```python
from build123d import *

# Parameters (mm, degrees)
F1_R          = 1.2
F2_DEPTH      = 2
F3_R          = 2
F4_W          = 4
F4_H          = 4.75
F5_DEPTH      = 9
F6_W          = 8.8
F6_H          = 2
F6_W_2        = 2
F6_H_2        = 6.5
F7_DEPTH      = 4
F8_R          = 0.8
F9_DEPTH      = 4
F10_T4_DEPTH  = 2
F10_S5_R      = 0.8
F10_T6_DEPTH  = 3
F10_T10_DEPTH = 6.5
F10_T15_DEPTH = 6.5
F10_T20_DEPTH = 2
F10_S21_R     = 0.8
F10_T22_DEPTH = 3
F10_T27_DEPTH = 6.5
F10_S29_R     = 0.8
F10_T30_DEPTH = 5
F10_T33_DEPTH = 4.5
F10_T40_DEPTH = 4.5
F10_T44_DEPTH = 6.5
F10_S46_R     = 0.8
F10_T47_DEPTH = 5
F10_T49_DEPTH = 6.5
F10_T51_DEPTH = 11.5
F11_W         = 2
F11_H         = 18
F12_DEPTH     = 12
F13_R         = 1.55
F13_R_2       = 0.8
F14_DEPTH     = 2
F15_R         = 0.8
F16_DEPTH     = 2
F18_W         = 20.8
F18_H         = 21.9
F19_DEPTH     = 0.4


# Not quite as in the source:
# - a fillet or chamfer that OpenCascade refuses, or shapes differently, is made with other operations: its cross-section is extruded or revolved along the edge and cut away or added
# - two fillets or chamfers of one size are made in one step


with BuildPart() as f2:
    # F1 (on Top) → F2 (new body)
    with BuildSketch(Plane.XY):
        with BuildLine():
            Line((-4.2895651858, 24.55), (-9.8, 24.55))
            Line((-9.8, 24.55), (-9.8, 6.55))
            Line((-9.8, 6.55), (-4.3, 6.55))
            Line((-4.3, 6.55), (-4.3, -5))
            ThreePointArc((-4.3, -5), (-3.4213203436, -7.1213203436), (-1.3, -8))
            Line((-1.3, -8), (22.7, -8))
            ThreePointArc((22.7, -8), (24.8213203436, -7.1213203436), (25.7, -5))
            Line((25.7, -5), (25.7, 6.55))
            Line((25.7, 6.55), (31.2, 6.55))
            Line((31.2, 6.55), (31.2, 24.55))
            Line((31.2, 24.55), (25.6895651858, 24.55))
            ThreePointArc((25.6895651858, 24.55), (24.7310096012, 26.5079402166), (22.7, 27.3))
            Line((22.7, 27.3), (-1.3, 27.3))
            ThreePointArc((-1.3, 27.3), (-3.3310096012, 26.5079402166), (-4.2895651858, 24.55))
        make_face()
        with Locations((-1.3, -5)):
            Circle(F1_R, mode=Mode.SUBTRACT)
        with Locations((22.7, -5)):
            Circle(F1_R, mode=Mode.SUBTRACT)
        with Locations((-1.3, 24.3)):
            Circle(F1_R, mode=Mode.SUBTRACT)
        with Locations((22.7, 24.3)):
            Circle(F1_R, mode=Mode.SUBTRACT)
    extrude(amount=F2_DEPTH)

    # F3
    f3_edges = [f2.edges().sort_by_distance(p)[0] for p in [
        (-4.289565, 24.55, 1),
        (-4.3, 6.55, 1),
        (25.7, 6.55, 1),
        (25.689565, 24.55, 1),
    ]]
    fillet(f3_edges, radius=F3_R)

    # F4 (on face) → F5 (join)
    with BuildSketch(Plane(origin=(0, 0, 0), x_dir=(1, 0, 0), z_dir=(0, 0, -1))):
        with Locations((13.8, 2.675)):
            Rectangle(F4_W, F4_H)
        with Locations((13.8, -23.975)):
            Rectangle(F4_W, F4_H)
    extrude(amount=F5_DEPTH)

    # F6 (on face) → F7 (join)
    with BuildSketch(Plane(origin=(0, 0, 0), x_dir=(1, 0, 0), z_dir=(0, 0, -1))):
        Polygon((-2.3, -18.3), (-0.3, -18.3), (-0.3, 0.3), (11.8, 0.3), (11.8, 2.3), (-2.3, 2.3), align=None)
        with Locations((7.4, -22.6)):
            Rectangle(F6_W, F6_H)
        with Locations((21.5, -3.25)):
            Rectangle(F6_W_2, F6_H_2)
    extrude(amount=F7_DEPTH)

    # F8 (on face) → F9 (cut, through all)
    with BuildSketch(Plane.YZ.offset(15.8)):
        with Locations((23.4, -5.75)):
            Circle(F8_R)
        with Locations((-2.1, -5.75)):
            Circle(F8_R)
    extrude(amount=-F9_DEPTH, mode=Mode.SUBTRACT)

    # F10: fillet of radius 1 on 10 edges, made by hand


with BuildPart() as f10_tool2:
    # F10_s3 → F10_t4 (new body)
    with BuildSketch(Plane.XZ.offset(0.3)):
        with BuildLine():
            ThreePointArc((11.8, -5), (11.5071067812, -4.2928932188), (10.8, -4))
            Line((10.8, -4), (11.8, -4))
            Line((11.8, -4), (11.8, -5))
        make_face()
    extrude(amount=F10_T4_DEPTH)

    # F10_s5 → F10_t6 (cut, symmetric)
    with BuildSketch(Plane.YZ.offset(11.3)):
        with Locations((-2.1, -5.75)):
            Circle(F10_S5_R)
    extrude(amount=F10_T6_DEPTH, both=True, mode=Mode.SUBTRACT)


with BuildPart() as f2_1:
    add(f2.part)

    # F10_t1: union F10_tool2
    add(f10_tool2.part)


with BuildPart() as f10_tool8:
    # F10_s9 → F10_t10 (new body)
    with BuildSketch(Plane.XY.offset(2.5)):
        with BuildLine():
            ThreePointArc((11.8, -3.3), (11.5071067812, -2.5928932188), (10.8, -2.3))
            Line((10.8, -2.3), (11.8, -2.3))
            Line((11.8, -2.3), (11.8, -3.3))
        make_face()
    extrude(amount=-F10_T10_DEPTH)

    split(bisect_by=Plane.XY.offset(2), keep=Keep.BOTTOM)


with BuildPart() as f2_2:
    add(f2_1.part)

    # F10_t7: union F10_tool8
    add(f10_tool8.part)


with BuildPart() as f10_tool13:
    # F10_s14 → F10_t15 (new body)
    with BuildSketch(Plane.XY.offset(2.5)):
        with BuildLine():
            ThreePointArc((11.8, 24.6), (11.5071067812, 23.8928932188), (10.8, 23.6))
            Line((10.8, 23.6), (11.8, 23.6))
            Line((11.8, 23.6), (11.8, 24.6))
        make_face()
    extrude(amount=-F10_T15_DEPTH)

    split(bisect_by=Plane.XY.offset(2), keep=Keep.BOTTOM)


with BuildPart() as f2_3:
    add(f2_2.part)

    # F10_t12: union F10_tool13
    add(f10_tool13.part)


with BuildPart() as f10_tool18:
    # F10_s19 → F10_t20 (new body)
    with BuildSketch(Plane.XZ.offset(-23.6)):
        with BuildLine():
            ThreePointArc((11.8, -5), (11.5071067812, -4.2928932188), (10.8, -4))
            Line((10.8, -4), (11.8, -4))
            Line((11.8, -4), (11.8, -5))
        make_face()
    extrude(amount=F10_T20_DEPTH)

    # F10_s21 → F10_t22 (cut, symmetric)
    with BuildSketch(Plane.YZ.offset(11.3)):
        with Locations((23.4, -5.75)):
            Circle(F10_S21_R)
    extrude(amount=F10_T22_DEPTH, both=True, mode=Mode.SUBTRACT)


with BuildPart() as f2_4:
    add(f2_3.part)

    # F10_t17: union F10_tool18
    add(f10_tool18.part)


with BuildPart() as f10_tool25:
    # F10_s26 → F10_t27 (new body)
    with BuildSketch(Plane.XY):
        with BuildLine():
            ThreePointArc((11.8, -3.3), (11.5071067812, -2.5928932188), (10.8, -2.3))
            Line((10.8, -2.3), (11.8, -2.3))
            Line((11.8, -2.3), (11.8, -3.3))
        make_face()
    extrude(amount=-F10_T27_DEPTH)

    split(bisect_by=Plane.XY.offset(-4), keep=Keep.BOTTOM)

    # F10_s29 → F10_t30 (cut, symmetric)
    with BuildSketch(Plane.YZ.offset(11.3)):
        with Locations((-2.1, -5.75)):
            Circle(F10_S29_R)
    extrude(amount=F10_T30_DEPTH, both=True, mode=Mode.SUBTRACT)


with BuildPart() as f10_tool31:
    # F10_s32 → F10_t33 (new body)
    with BuildSketch(Plane.XZ.offset(0.3)):
        with BuildLine():
            ThreePointArc((11.8, -5), (11.5071067812, -4.2928932188), (10.8, -4))
            Line((10.8, -4), (11.8, -4))
            Line((11.8, -4), (11.8, -5))
        make_face()
    extrude(amount=F10_T33_DEPTH)

    split(bisect_by=Plane.XZ.offset(2.3), keep=Keep.TOP)


with BuildPart() as f10_tool25_1:
    add(f10_tool25.part)

    # F10_t35: intersect F10_tool31
    add(f10_tool31.part, mode=Mode.INTERSECT)


with BuildPart() as f2_5:
    add(f2_4.part)

    # F10_t23: union F10_tool25
    add(f10_tool25_1.part)


with BuildPart() as f10_tool38:
    # F10_s39 → F10_t40 (new body)
    with BuildSketch(Plane.XZ.offset(-26.1)):
        with BuildLine():
            ThreePointArc((11.8, -5), (11.5071067812, -4.2928932188), (10.8, -4))
            Line((10.8, -4), (11.8, -4))
            Line((11.8, -4), (11.8, -5))
        make_face()
    extrude(amount=F10_T40_DEPTH)

    split(bisect_by=Plane.XZ.offset(-23.6), keep=Keep.BOTTOM)


with BuildPart() as f10_tool42:
    # F10_s43 → F10_t44 (new body)
    with BuildSketch(Plane.XY):
        with BuildLine():
            ThreePointArc((11.8, 24.6), (11.5071067812, 23.8928932188), (10.8, 23.6))
            Line((10.8, 23.6), (11.8, 23.6))
            Line((11.8, 23.6), (11.8, 24.6))
        make_face()
    extrude(amount=-F10_T44_DEPTH)

    split(bisect_by=Plane.XY.offset(-4), keep=Keep.BOTTOM)

    # F10_s46 → F10_t47 (cut, symmetric)
    with BuildSketch(Plane.YZ.offset(11.3)):
        with Locations((23.4, -5.75)):
            Circle(F10_S46_R)
    extrude(amount=F10_T47_DEPTH, both=True, mode=Mode.SUBTRACT)


with BuildPart() as f10_tool38_1:
    add(f10_tool38.part)

    # F10_t48: intersect F10_tool42
    add(f10_tool42.part, mode=Mode.INTERSECT)


with BuildPart() as f2_6:
    add(f2_5.part)

    # F10_t36: union F10_tool38
    add(f10_tool38_1.part)

    # F10_s50 → F10_t49 (cut)
    with BuildSketch(Plane.XY.offset(-6.5)):
        with BuildLine():
            ThreePointArc((-1.3, -2.3), (-2.0071067812, -2.0071067812), (-2.3, -1.3))
            Line((-2.3, -1.3), (-2.3, -2.3))
            Line((-2.3, -2.3), (-1.3, -2.3))
        make_face()
        with BuildLine():
            ThreePointArc((-2.3, 17.3), (-2.0071067812, 18.0071067812), (-1.3, 18.3))
            Line((-1.3, 18.3), (-2.3, 18.3))
            Line((-2.3, 18.3), (-2.3, 17.3))
        make_face()
        with BuildLine():
            ThreePointArc((3, 22.6), (3.2928932188, 23.3071067812), (4, 23.6))
            Line((4, 23.6), (3, 23.6))
            Line((3, 23.6), (3, 22.6))
        make_face()
        with BuildLine():
            ThreePointArc((21.5, 0), (22.2071067812, 0.2928932188), (22.5, 1))
            Line((22.5, 1), (22.5, 0))
            Line((22.5, 0), (21.5, 0))
        make_face()
    extrude(amount=F10_T49_DEPTH, mode=Mode.SUBTRACT)

    # F10_s52 → F10_t51 (cut)
    with BuildSketch(Plane.XY.offset(-11.5)):
        with BuildLine():
            ThreePointArc((11.8, 25.35), (12.0928932188, 26.0571067812), (12.8, 26.35))
            Line((12.8, 26.35), (11.8, 26.35))
            Line((11.8, 26.35), (11.8, 25.35))
        make_face()
        with BuildLine():
            ThreePointArc((12.8, -5.05), (12.0928932188, -4.7571067812), (11.8, -4.05))
            Line((11.8, -4.05), (11.8, -5.05))
            Line((11.8, -5.05), (12.8, -5.05))
        make_face()
    extrude(amount=F10_T51_DEPTH, mode=Mode.SUBTRACT)

    # F11 (on face) → F12 (join)
    with BuildSketch(Plane(origin=(0, 0, 0), x_dir=(1, 0, 0), z_dir=(0, 0, -1))):
        with Locations((-8.8, -15.55)):
            Rectangle(F11_W, F11_H)
        with Locations((30.2, -15.55)):
            Rectangle(F11_W, F11_H)
    extrude(amount=F12_DEPTH)

    # F13 (on face) → F14 (cut, through all)
    with BuildSketch(Plane(origin=(-9.8, 0, 0), x_dir=(0, -1, 0), z_dir=(-1, 0, 0))):
        with Locations((-15.55, -5.75)):
            Circle(F13_R)
        with Locations((-21.55, -5.75)):
            Circle(F13_R_2)
        with Locations((-9.55, -5.75)):
            Circle(F13_R_2)
        with BuildLine():
            ThreePointArc((-22.0259169235, -12), (-23.8951558497, -9.1202186642), (-24.55, -5.75))
            Line((-24.55, -5.75), (-24.55, -12))
            Line((-24.55, -12), (-22.0259169235, -12))
        make_face()
        with BuildLine():
            ThreePointArc((-6.55, -5.75), (-7.2048441503, -9.1202186642), (-9.0740830765, -12))
            Line((-9.0740830765, -12), (-6.55, -12))
            Line((-6.55, -12), (-6.55, -5.75))
        make_face()
    extrude(amount=-F14_DEPTH, mode=Mode.SUBTRACT)

    # F15 (on face) → F16 (cut, through all)
    with BuildSketch(Plane.YZ.offset(31.2)):
        with BuildLine():
            ThreePointArc((24.55, -1.2876575658), (22.9160115829, -3.4891181199), (20.3357142857, -2.562612547))
            ThreePointArc((20.3357142857, -2.562612547), (15.55, 0), (10.7642857143, -2.562612547))
            ThreePointArc((10.7642857143, -2.562612547), (8.1839884171, -3.4891181199), (6.55, -1.2876575658))
            Line((6.55, -1.2876575658), (6.55, -12))
            Line((6.55, -12), (24.55, -12))
            Line((24.55, -12), (24.55, -1.2876575658))
        make_face()
        with Locations((8.85, -1.2876575658)):
            Circle(F15_R)
        with Locations((22.25, -1.2876575658)):
            Circle(F15_R)
    extrude(amount=-F16_DEPTH, mode=Mode.SUBTRACT)

    # F18 (on face) → F19 (cut)
    with BuildSketch(Plane(origin=(0, 0, 0), x_dir=(1, 0, 0), z_dir=(0, 0, -1))):
        with Locations((10.1, -10.65)):
            Rectangle(F18_W, F18_H)
    extrude(amount=-F19_DEPTH, mode=Mode.SUBTRACT)


solid = f2_6.part
```
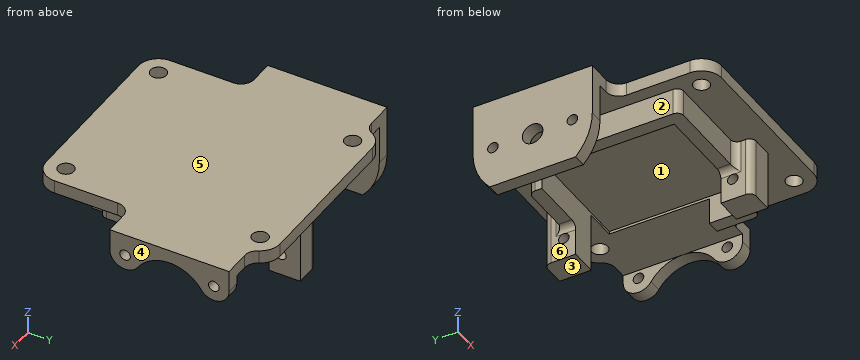
Geometry: final body of the model. Coordinates: model frame, mm. Face numbers are marked on the shaded views. A direction names the side the tool comes from. Give positions to 0.01 mm unless a question says otherwise; leave off trailing zeros. Write each loop counter-clockwise with the first axis right and the second up, starting at its lowest first coordinate (ties: lowest second). Pieces come first, ordered by that corner, then holes.
1. Draft query along X for the marked faces 4, 5 and 6. Return one class per face: released by +X, released by -X, zero draft, split by the parting line, or undercut.
2. Section query C-C, the plane y = 12.5. Return loops of the section in (x, z).
3. Line query: probe 1 along Y at (x, z) = (-1.3, 0.55); probe 2 along Y at (x, z) = (13, -5.75); probe 3 along X at (y, z) = (1, -3.5). Output: solid intervals per line, ascending.
4. Reachability of the marked faces 1, 2 and 3 from +Z, -Z, +X, -X, +Y, -Y: full face, straight path, thin tool, end or side. Return the list, or none.
5. Section query B-B, the plane y = 5. Return loops of the section in (x, z).
6. Section query A-A, the plane x = 1. Return loops of the section in (y, z).
7. Pin query (flat end, axial travel): P1, Ø8, axis at y = 2, z = -6.5, coming from the +X side; P2, Ø6, axis at x = -5, z = -9.5, coming from the -Y side; P3, Ø1.1, axis at x = 21, z = -3, coming from the -Y side. Return the tip coordinate at first contact, or that it passes through.
Computed:
1. face 4: released by +X
1. face 5: zero draft
1. face 6: undercut
2. outline: (-9.8, -12) - (-7.8, -12) - (-7.8, 0) - (-2.3, 0) - (-2.3, -4) - (-0.3, -4) - (-0.3, 0.4) - (20.5, 0.4) - (20.5, 0) - (29.2, 0) - (29.2, -0.88) - (31.2, -0.88) - (31.2, 2) - (-9.8, 2) - close
3. probe 1: y = -8 to -6.2, -3.8 to 23.1, 25.5 to 27.3
3. probe 2: y = -5.05 to -2.9, -1.3 to -0.3, 21.6 to 22.6, 24.2 to 26.35
3. probe 3: x = -2.3 to -0.3, 20.5 to 22.5
4. face 1: -Z
4. face 2: -Z, +Y, -Y
4. face 3: -Z, +X, +Y, -Y
5. outline: (-4.35, 0) - (-2.3, 0) - (-2.3, -4) - (-0.3, -4) - (-0.3, 0.4) - (20.5, 0.4) - (20.5, -4) - (22.5, -4) - (22.5, 0) - (25.75, 0) - (25.75, 2) - (-4.35, 2) - close
6. outline: (-8, 0) - (-2.3, 0) - (-2.3, -4) - (-0.3, -4) - (-0.3, 0.4) - (21.6, 0.4) - (21.6, 0) - (27.3, 0) - (27.3, 2) - (-8, 2) - close
7. P1: stops at x = 22.5
7. P2: stops at y = 6.96
7. P3: stops at y = 0
